For this review, take the finished solid that the model builds, in its own axes (mm). A direction names the side the tool comes from. Round coordinates to 2 decimals unless told otherwise and drop trailing zeros. Loops run counter-clockwise (first coordinate to the right, second up) from the corner with the lowest first, then second, coordinate; pieces in that order, holes last.
1) Take a section at D-D (y = 384.5). State the section outline as (x, z) points, then the cut area to 3 significant figures.
2) Take a section at C-C (z = 61). State the section outline as (x, y) points, then the cut area to 3 significant figures.
3) Take a section at B-B (x = -66). State the section outline as (y, z) points, then the cut area to 3 significant figures.
4) Wall thickness on L1, parallel to X at y = 241, z = 35; L2, parallel to X at y = 749.5, z = 44.5; L3, parallel to Y at x = -102.5, z = 8.5: over which ranges is each line inside the solid? List them lowest first.
5) Tool access review of faces 4 (the flat face through (-100.084, 241, 35)), 5 (the flat face through (-114, 469, 0)), 6 (the flat face through (-100.084, 708, 35)): name each direction out of +Z, -Z, +X, -X, +Y, -Y from which nothing blocks a thin tool from reaching the whole face with its end or side.
6) Take a section at A-A (z = 35). State the section outline as (x, y) points, then the cut area to 3 significant figures.
7) Mouldability with a two-part tool opening along Z and no side actions: class faces 1 (the cylindrical face through (-49.38, 204.56, 48.52)), 2 (the flat face through (-0.084, 238, 27)), 3 (the flat face through (-114, 469, 70)) as pulls with the +Z half, pulls with the -Z half, needs draft (parallel to the pull), parting line crosses it, or undercut.
8) Insertion check: pin 1 (1 mm diameter, centred on y = 487, z = 56.5, fed in from +X); pin 2 (12 mm diameter, centred on x = -113.5, y = 684, fed in from -Z); pin 3 (10 mm diameter, centred on y = 490, z = 20.5, fed in from -X); pin 4 (4 mm diameter, centred on y = 233.5, z = 27.5, fed in from -X). Each pin has a flat end and moves straight along its axis. Give the tip position at first contact, or say it passes through.
```python
from build123d import *

# Parameters (mm, degrees)
BOSS_EXTRUDE1_DEPTH = 70
SKETCH2_R           = 20
CUT_EXTRUDE1_DEPTH  = 192
CUT_EXTRUDE2_DEPTH  = 192
CUT_EXTRUDE3_DEPTH  = 192


with BuildPart() as part:
    # Sketch1 → Boss-Extrude1 (new body)
    with BuildSketch(Plane.XY):
        with BuildLine():
            Line((-100.084321869, 339.298857864), (-100.084321869, 139.298857864))
            Line((-100.084321869, 139.298857864), (-0.084321869, 139.298857864))
            Line((-0.084321869, 139.298857864), (-0.084321869, 339.298857864))
            Line((-0.084321869, 339.298857864), (-100.084321869, 639.298857864))
            Line((-100.084321869, 639.298857864), (-100.084321869, 779.298857864))
            ThreePointArc((-100.084321869, 779.298857864), (-103.013254057, 786.369925676), (-110.084321869, 789.298857864))
            Line((-110.084321869, 789.298857864), (-215.084321869, 789.298857864))
            ThreePointArc((-215.084321869, 789.298857864), (-222.155389681, 786.369925676), (-225.084321869, 779.298857864))
            Line((-225.084321869, 779.298857864), (-225.084321869, 639.298857864))
            Line((-225.084321869, 639.298857864), (-100.084321869, 339.298857864))
        make_face()
    extrude(amount=BOSS_EXTRUDE1_DEPTH)

    # Sketch2 → Cut-Extrude1 (cut)
    with BuildSketch(Plane(origin=(-0.084321869, 0, 0), x_dir=(0, 0, -1), z_dir=(1, 0, 0))):
        with Locations(Location((-35, 289.298857864, 0), (0, 0, 90))):
            Circle(SKETCH2_R)
        with Locations(Location((-35, 219.298857864, 0), (0, 0, 90))):
            Circle(SKETCH2_R)
    extrude(amount=-CUT_EXTRUDE1_DEPTH, mode=Mode.SUBTRACT)

    # Sketch3 → Cut-Extrude2 (cut)
    with BuildSketch(Plane.XY.offset(70)):
        with BuildLine():
            Line((-225.084321869, 769.298857864), (-225.084321869, 749.298857864))
            Line((-225.084321869, 749.298857864), (-225.084321869, 729.298857864))
            ThreePointArc((-225.084321869, 729.298857864), (-205.084321869, 749.298857864), (-225.084321869, 769.298857864))
        make_face()
        with BuildLine():
            Line((-225.084321869, 689.298857864), (-225.084321869, 669.298857864))
            ThreePointArc((-225.084321869, 669.298857864), (-205.084321869, 689.298857864), (-225.084321869, 709.298857864))
            Line((-225.084321869, 709.298857864), (-225.084321869, 689.298857864))
        make_face()
    extrude(amount=-CUT_EXTRUDE2_DEPTH, mode=Mode.SUBTRACT)

    # Sketch4 → Cut-Extrude3 (cut)
    with BuildSketch(Plane.XY.offset(70)):
        with BuildLine():
            Line((-218.417655203, 730.442677032), (-225.084321869, 729.298857864))
            Line((-225.084321869, 729.298857864), (-225.084321869, 721.014586617))
            ThreePointArc((-225.084321869, 721.014586617), (-223.249287678, 726.788089308), (-218.417655203, 730.442677032))
        make_face()
        with BuildLine():
            Line((-225.084321869, 717.583129111), (-225.084321869, 709.298857864))
            Line((-225.084321869, 709.298857864), (-218.417655203, 708.155038696))
            ThreePointArc((-218.417655203, 708.155038696), (-223.249287678, 711.80962642), (-225.084321869, 717.583129111))
        make_face()
        with BuildLine():
            Line((-218.417655203, 670.442677032), (-225.084321869, 669.298857864))
            Line((-225.084321869, 669.298857864), (-225.084321869, 661.014586617))
            ThreePointArc((-225.084321869, 661.014586617), (-223.249287678, 666.788089308), (-218.417655203, 670.442677032))
        make_face()
        with BuildLine():
            Line((-225.084321869, 777.583129111), (-225.084321869, 769.298857864))
            Line((-225.084321869, 769.298857864), (-218.417655203, 768.155038696))
            ThreePointArc((-218.417655203, 768.155038696), (-223.249287678, 771.80962642), (-225.084321869, 777.583129111))
        make_face()
    extrude(amount=-CUT_EXTRUDE3_DEPTH, mode=Mode.SUBTRACT)


solid = part.part
```
Response:
1. outline: (-118.92, 0) - (-15.15, 0) - (-15.15, 70) - (-118.92, 70) - close
1. area: 7,260 mm2
2. outline: (-225.08, 639.3) - (-100.08, 339.3) - (-100.08, 139.3) - (-0.08, 139.3) - (-0.08, 339.3) - (-100.08, 639.3) - (-100.08, 779.3) arc R10 ccw to (-110.08, 789.3) - (-215.08, 789.3) arc R10 ccw to (-225.08, 779.3) - (-225.08, 777.58) arc R10 ccw to (-218.42, 768.16) arc R20 cw to (-218.42, 730.44) arc R10 ccw to (-225.08, 721.01) - (-225.08, 717.58) arc R10 ccw to (-218.42, 708.16) arc R20 cw to (-218.42, 670.44) arc R10 ccw to (-225.08, 661.01) - close
2. area: 71,200 mm2
3. outline: (139.3, 0) - (537.05, 0) - (537.05, 70) - (139.3, 70) - close; hole circle Ø40 at (219.3, 35); hole circle Ø40 at (289.3, 35)
3. area: 25,300 mm2
4. L1: x = -100.08 to -0.08
4. L2: x = -205.09 to -100.08
4. L3: y = 345.1 to 785.82
5. face 4: +Z, -Z, -X, -Y
5. face 5: -Z, +X, -X, +Y, -Y
5. face 6: +Z, -Z, +X, +Y
6. outline: (-225.08, 639.3) - (-100.08, 339.3) - (-100.08, 309.3) - (-0.08, 309.3) - (-0.08, 339.3) - (-100.08, 639.3) - (-100.08, 779.3) arc R10 ccw to (-110.08, 789.3) - (-215.08, 789.3) arc R10 ccw to (-225.08, 779.3) - (-225.08, 777.58) arc R10 ccw to (-218.42, 768.16) arc R20 cw to (-218.42, 730.44) arc R10 ccw to (-225.08, 721.01) - (-225.08, 717.58) arc R10 ccw to (-218.42, 708.16) arc R20 cw to (-218.42, 670.44) arc R10 ccw to (-225.08, 661.01) - close; (-100.08, 139.3) - (-0.08, 139.3) - (-0.08, 199.3) - (-100.08, 199.3) - close; (-100.08, 239.3) - (-0.08, 239.3) - (-0.08, 269.3) - (-100.08, 269.3) - close
6. area: 63,200 mm2
7. face 1: undercut
7. face 2: needs draft
7. face 3: pulls with the +Z half
8. pin 1: stops at x = -49.15
8. pin 2: stops at z = 0
8. pin 3: stops at x = -164.96
8. pin 4: passes through
